Design review of the part built by this model. Coordinates are the model's own, in mm. A direction names the side the tool comes from. Coordinates: 2 decimals unless noted, no trailing zeros. Write item = value, one per line.
```python
from build123d import *

# Parameters (mm, degrees)
BOSS_EXTRUDE1_DEPTH = 5.8
SKETCH3_W           = 4.2
SKETCH3_H           = 12
CUT_EXTRUDE1_DEPTH  = 6.35
SKETCH4_R           = 1.55
CUT_EXTRUDE2_DEPTH  = 6.8
SKETCH5_R           = 1.55
CUT_EXTRUDE3_DEPTH  = 6.8


with BuildPart() as part:
    # Sketch2 → Boss-Extrude1 (new body)
    with BuildSketch(Plane.XY):
        with BuildLine():
            Line((163, 44.2), (10, 44.2))
            ThreePointArc((10, 44.2), (2.928932188, 41.271067812), (0, 34.2))
            Line((0, 34.2), (0, -34.2))
            ThreePointArc((0, -34.2), (2.928932188, -41.271067812), (10, -44.2))
            Line((10, -44.2), (163, -44.2))
            ThreePointArc((163, -44.2), (170.071067812, -41.271067812), (173, -34.2))
            Line((173, -34.2), (173, 34.2))
            ThreePointArc((173, 34.2), (170.071067812, 41.271067812), (163, 44.2))
        make_face()
    extrude(amount=BOSS_EXTRUDE1_DEPTH)

    # Sketch3 → Cut-Extrude1 (cut)
    with BuildSketch(Plane.XY.offset(5.8)):
        with Locations((165.5, 6)):
            Rectangle(SKETCH3_W, SKETCH3_H)
    extrude(amount=-CUT_EXTRUDE1_DEPTH, mode=Mode.SUBTRACT)

    # Sketch4 → Cut-Extrude2 (cut, through all)
    with BuildSketch(Plane.XY.offset(5.8)):
        with Locations((17, 32.5)):
            Circle(SKETCH4_R)
        with Locations((17, 18.5)):
            Circle(SKETCH4_R)
        with Locations((17, -18.5)):
            Circle(SKETCH4_R)
        with Locations((17, -32.5)):
            Circle(SKETCH4_R)
    extrude(amount=-CUT_EXTRUDE2_DEPTH, mode=Mode.SUBTRACT)

    # Sketch5 → Cut-Extrude3 (cut, through all)
    with BuildSketch(Plane.XY.offset(5.8)):
        with Locations((165.5, 16.45)):
            Circle(SKETCH5_R)
        with Locations((165.5, -9.55)):
            Circle(SKETCH5_R)
    extrude(amount=-CUT_EXTRUDE3_DEPTH, mode=Mode.SUBTRACT)


solid = part.part
```
(1) Insertion check: pin 1 (2 mm diameter, centred on x = 166, z = 2.5, fed in from +Y). The pin has a flat end and moves straight along its axis. Give the tip position at first contact, or say it passes through.
Report:
pin_1 = 44
(2) For L1, parallel to Y at x = 17, z = 2.7; L2, parallel to X at y = 5, z = 0.3; L3, parallel to Y at x = 165.5, z = 4.2, list the stretches that pass through material, from the lowest coordinate up.
Report:
L1 = -44.2 to -34.05, -30.95 to -20.05, -16.95 to 16.95, 20.05 to 30.95, 34.05 to 44.2
L2 = 0 to 163.4, 167.6 to 173
L3 = -43.88 to -11.1, -8 to 0, 12 to 14.9, 18 to 43.88
(3) The part is to be moulded in two halves that separate along Y. For faces 3 (the cylindrical face through (2.85, -41.19, 2.86)), 4 (the flat face through (163.4, 6, 3)), 5 (the flat face through (85, 1, 0)), 6 (the cylindrical face through (163.95, -9.48, 2.94)), say which applies: released by +Y, released by -Y, zero draft, split by the parting line, or undercut.
Report:
face_3 = released by -Y
face_4 = undercut
face_5 = zero draft
face_6 = undercut
(4) For faces 1 (the flat face through (85, -44.2, 3)), 2 (the flat face through (167.6, 6, 3)), list the 3-axis set-ups (+Z, -Z, +X, -X, +Y, -Y) from which the entire face can be reached by the end or side of a thin tool; tool diameter is ignored.
Report:
face_1 = +Z, -Z, +X, -X, -Y
face_2 = +Z, -Z
